from build123d import *

# Parameters (mm, degrees)
SKETCH_W     = 162
SKETCH_H     = 31.5
PAD_DEPTH    = 3
CHAMFER_SIZE = 2.5


with BuildPart() as part:
    # Sketch → Pad (new body)
    with BuildSketch(Plane.XY):
        with Locations((81, -15.75)):
            Rectangle(SKETCH_W, SKETCH_H)
    extrude(amount=PAD_DEPTH)

    # Chamfer
    chamfer_edges = [part.edges().sort_by_distance(p)[0] for p in [
        (81, -31.5, 3),
        (81, 0, 3),
    ]]
    chamfer(chamfer_edges, length=CHAMFER_SIZE)


solid = part.part
Check sheet for the modelled part. Datum: model origin and axes. Units: mm. Round coordinates to 2 decimals unless told otherwise and drop trailing zeros. Write each loop counter-clockwise with the first axis right and the second up, starting at its lowest first coordinate (ties: lowest second). Pieces come first, ordered by that corner, then holes. Notation, with made-up numbers: (-38.75, -3) - (-21.75, -3) arc R18 ccw to (-21.75, 6) - close; hole circle Ø2 at (-28.75, 70.25). An arc over 180 degrees is marked (long way). Return JSON: item names as keys, results as strings.
Q1. Cross-section at B-B (z = 1.1). Record the boundary of the cut face in (x, y).
Returned:
{"outline": "(0, -30.9) - (162, -30.9) - (162, -0.6) - (0, -0.6) - close"}
Q2. Depth check by flat-ended pin: P1, Ø1.5, axis at y = -17.5, z = 1, coming from the -X side. Enter the tip coordinate at first touch or a pass-through.
Returned:
{"P1": "stops at x = 0"}
Q3. Scan lines: L1, parallel to Y at x = 28.5, z = 2.25; L2, parallel to Y at x = 94, z = 2.95; L3, parallel to Z at x = 102, y = -0.5. Record each from-to range of solid material in increasing order. Write a range as from..to.
Returned:
{"L1": "y = -29.75..-1.75", "L2": "y = -29.05..-2.45", "L3": "z = 0..1"}
Q4. Cross-section at A-A (x = 87.5). Record the boundary of the cut face in (y, z), then the cut area to 4 significant figures.
Returned:
{"outline": "(-31.5, 0) - (0, 0) - (0, 0.5) - (-2.5, 3) - (-29, 3) - (-31.5, 0.5) - close", "area": "88.25 mm²"}
